Autodesk Inventor part; units mm, degrees
ref_plane "YZ Plane" through (0, 0, 0) normal (1, 0, 0) x (0, 1, 0)
ref_plane "XZ Plane" through (0, 0, 0) normal (0, 1, 0) x (-1, 0, 0)
ref_plane "XY Plane" through (0, 0, 0) normal (0, 0, 1) x (1, 0, 0)
sketch "Sketch1" plane through (0, 0, 0) normal (0, 0, 1) x (1, 0, 0)
  circle A0 centre (0, 0) radius 28
  dimension "d0" = 56
extrude "Extrusion1" add sketch "Sketch1" along normal blind 5
sketch "Sketch2" plane through (0, 0, 5) normal (0, 0, 1) x (1, 0, 0)
  line L0 (0, 0) -> (30, 0) construction
  line L1 (30, 0) -> (30, 30) construction
  line L2 (30, 30) -> (0, 30) construction
  line L3 (0, 30) -> (0, 0) construction
  circle A0 centre (0, 0) radius 30 construction
  circle A1 centre (30, 30) radius 30 construction
  circle A2 centre (0, 0) radius 12.4264 construction
  circle A3 centre (30, 30) radius 25
  circle A4 centre (0, 0) radius 4
  line L4 (12.4264, 0) -> (30, 0) construction
  line L5 (12.4264, -3) -> (30, -3)
  line L6 (30, 3) -> (12.4264, 3)
  arc A5 (12.4264, 3) -> (12.4264, -3) centre (12.4264, 0) ccw
  arc A6 (30, -3) -> (30, 3) centre (30, 0) ccw
  point P0 (21.2132, 0)
  dimension "d5" = 60
  dimension "d3" = 30
  dimension "d4" = 30
  dimension "d6" = 60
  dimension "d7" = 50
  dimension "d8" = 8
  dimension "d9" = 6
extrude "Extrusion2" cut sketch "Sketch2" against normal blind 5
pattern_circular "Circular Pattern1" count 4 over 360 about axis through (0, 0, 5) along (0, 0, -1) of "Extrusion2"
properties part number "Geneva_driven"
Geometry check sheet. Reference: the model listing, model coordinates, mm. A direction names the side the tool comes from. Give positions to 0.01 mm unless a question says otherwise; leave off trailing zeros. Order: outer loops, then holes, each group sorted by start corner. A loop starts at its lowest first (then second) coordinate and runs counter-clockwise, first axis right, second up. Notation, with made-up numbers: (-31, 28.5) - (26, 28.5) arc R14 cw to (26, 53.5) - close; hole circle Ø1 at (-10, -39). An arc over 180 degrees is marked (long way). Use one line per item in the form item = value.
1) Sectioned sample at D-D (y = 6). Record the boundary of the cut face in (x, z), and give its area (3 significant figures).
Working result:
outline = (-23, 0) - (23, 0) - (23, 5) - (-23, 5) - close
area = 230 mm^2
2) Material ranges on probe 1 along X at (y, z) = (0, 3.05); probe 2 along Y at (x, z) = (10, 3.6), recorded low to high. Write a range as from..to.
Working result:
probe_1 = -9.43..-4, 4..9.43
probe_2 = -15..-1.76, 1.76..15
3) Depth check by flat-ended pin: pin 1 Ø2 at (y, z) = (-9, 4) entering from -X; pin 2 Ø6.5 at (x, y) = (0, 0) entering from -Z; pin 3 Ø2.5 at (y, z) = (-22.5, 2.5) entering from -X; pin 4 Ø2.5 at (y, z) = (-21, 3) entering from +X. Enter the tip coordinate at first touch or a pass-through.
Working result:
pin_1 = -18.13
pin_2 = through
pin_3 = -6.58
pin_4 = 7.2
4) Access from +Z, -Z, +X, -X, +Y, -Y to the whole of each face (thin tool, end or side, straight path). Record for faces 5 (the face through (20, -3, 3)), 6 (the face through (3, -20, 3)), 7 (the face through (-3, 20, 3)), 8 (the face through (-20, -3, 3)).
Working result:
face_5 = +Z, -Z, +X
face_6 = +Z, -Z, -Y
face_7 = +Z, -Z, +Y
face_8 = +Z, -Z, -X
5) Sectioned sample at A-A (x = 0). Record the boundary of the cut face in (y, z).
Working result:
outline = (-9.43, 0) - (-4, 0) - (-4, 5) - (-9.43, 5) - close; (4, 0) - (9.43, 0) - (9.43, 5) - (4, 5) - close
6) Draft check along Y on faces 1 (the face through (-3, -20, 3)), 2 (the face through (-9.427, -0.066, 2.535)), 3 (the face through (20, 3, 3)), 4 (the face through (12.153, 12.493, 2.535)). Enter one of: released by +Y, released by -Y, zero draft, split by the parting line, or undercut.
Working result:
face_1 = zero draft
face_2 = undercut
face_3 = undercut
face_4 = released by +Y
7) Sectioned sample at B-B (z = 1.95). Record the boundary of the cut face in (x, y).
Working result:
outline = (-27.84, -3) arc R28 ccw to (-27.53, -5.12) arc R25 cw to (-5.12, -27.53) arc R28 ccw to (-3, -27.84) - (-3, -12.43) arc R3 cw to (3, -12.43) - (3, -27.84) arc R28 ccw to (5.12, -27.53) arc R25 cw to (27.53, -5.12) arc R28 ccw to (27.84, -3) - (12.43, -3) arc R3 cw to (12.43, 3) - (27.84, 3) arc R28 ccw to (27.53, 5.12) arc R25 cw to (5.12, 27.53) arc R28 ccw to (3, 27.84) - (3, 12.43) arc R3 cw to (-3, 12.43) - (-3, 27.84) arc R28 ccw to (-5.12, 27.53) arc R25 cw to (-27.53, 5.12) arc R28 ccw to (-27.84, 3) - (-12.43, 3) arc R3 cw to (-12.43, -3) - close; hole circle Ø8 at (0, 0)
